Here's how the part is built. I have some questions about the finished solid (model axes, mm). A direction names the side the tool comes from. Round coordinates to 2 decimals unless told otherwise and drop trailing zeros. Order: outer loops, then holes, each group sorted by start corner. A loop starts at its lowest first (then second) coordinate and runs counter-clockwise, first axis right, second up. Notation, with made-up numbers: (29, 25) -> (68, 25) arc R34 cw to (68, 56) -> close; hole circle Ø4 at (-24, -37). An arc over 180 degrees is marked (long way). Use a Markdown table: item, result. Add a question column.
(1) I want a section at A-A, the plane y = 8.75. Please give me the cut outline in (x, z).
(2) Thinking about a two-plate mould opening in X: for faces 1 (the face through (-22, 6.65, 11)), 2 (the face through (13.14, 2.22, -10.1)), 3 (the face through (13.75, 9.69, 11.14)), which applies, pulls with the +X half, pulls with the -X half, needs draft (parallel to the pull), parting line crosses it, or undercut?
(3) I'm going to push flat-ended pins straight in: P1, Ø1.2, axis at y = 8.5, z = 4.5, coming from the +X side; P2, Ø1.8, axis at x = 10, z = 33, coming from the -Y side; P3, Ø2, axis at y = 10, z = 31.5, coming from the -X side. Where does each tip first touch, or does it pass through?
(4) I want a section at C-C, the plane x = -6. Please give me the cut outline in (y, z).
(5) On a 3-axis mill with a long thin cutter (end or side, diameter ignored), from which of +Z, -Z, +X, -X, +Y, -Y can I reach the whole of each face in a straight line? I mean faces 4 (the face through (11, 2, 35)), 5 (the face through (-18.75, 10, 4)), 6 (the face through (18.75, 10, 4)). Say none if no direction works.
(6) If I drill on probe 1 along X at (y, z) = (9.25, 32); probe 2 along X at (y, z) = (2, 11.25); probe 3 along Z at (x, y) = (-9.5, 2), over which ranges is the centre line in solid material (lowest first)?
(7) I want a section at B-B, the plane y = 1.25. Give the number of separate pieces and of enclosed holes in the cut face, then the cut area to 3 significant figures.
(8) I want a section at D-D, the plane x = 20. Please give me the cut outline in (y, z), then the cut area to 3 significant figures.
from build123d import *

# Parameters (mm, degrees)
SCHIZZO3_R                   = 2.25
ESTRUSIONE_ESTRUSIONE1_DEPTH = 12.65
SCHIZZO1_R                   = 3
TAGLIO_ESTRUSIONE1_DEPTH     = 4.5
SCHIZZO4_R                   = 10.75
SCHIZZO4_R_2                 = 1.45
TAGLIO_ESTRUSIONE2_DEPTH     = 48.529438246
SCHIZZO6_R                   = 5
TAGLIO_ESTRUSIONE3_DEPTH     = 6
SCHIZZO7_W                   = 16
SCHIZZO7_H                   = 77
TAGLIO_ESTRUSIONE4_DEPTH     = 6


with BuildPart() as part:
    # Schizzo3 → Estrusione-Estrusione1 (new body)
    with BuildSketch(Plane(origin=(0, 0, 0), x_dir=(1, 0, 0), z_dir=(0, 1, 0))):
        with BuildLine():
            Line((-24.75, 2.881082761), (-24.75, -25.381082761))
            ThreePointArc((-24.75, -25.381082761), (0, -39.75), (24.75, -25.381082761))
            Line((24.75, -25.381082761), (24.75, 2.881082761))
            ThreePointArc((24.75, 2.881082761), (0, 17.25), (-24.75, 2.881082761))
        make_face()
        with Locations(Location((-18.75, 2.75, 0), (0, 0, 270))):
            Circle(SCHIZZO3_R, mode=Mode.SUBTRACT)
        with Locations(Location((18.75, 2.75, 0), (0, 0, 90))):
            Circle(SCHIZZO3_R, mode=Mode.SUBTRACT)
        with Locations(Location((18.75, -25.25, 0), (0, 0, 270))):
            Circle(SCHIZZO3_R, mode=Mode.SUBTRACT)
        with Locations(Location((-18.75, -25.25, 0), (0, 0, 90))):
            Circle(SCHIZZO3_R, mode=Mode.SUBTRACT)
        with Locations(Location((-18.75, -11.25, 0), (0, 0, 270))):
            Circle(SCHIZZO3_R, mode=Mode.SUBTRACT)
        with Locations(Location((18.75, -11.25, 0), (0, 0, 90))):
            Circle(SCHIZZO3_R, mode=Mode.SUBTRACT)
    extrude(amount=ESTRUSIONE_ESTRUSIONE1_DEPTH)

    # Schizzo1 → Taglio-Estrusione1 (cut)
    with BuildSketch(Plane(origin=(0, 0, 0), x_dir=(1, 0, 0), z_dir=(0, 1, 0))):
        with Locations(Location((-11, -32, 0), (0, 0, 270))):
            Circle(SCHIZZO1_R)
        with Locations(Location((11, -32, 0), (0, 0, 90))):
            Circle(SCHIZZO1_R)
        with BuildLine():
            Line((-14, 8), (-14, -8))
            ThreePointArc((-14, -8), (-13.121320344, -10.121320344), (-11, -11))
            Line((-11, -11), (0, -11))
            Line((0, -11), (11, -11))
            ThreePointArc((11, -11), (13.121320344, -10.121320344), (14, -8))
            Line((14, -8), (14, 8))
            ThreePointArc((14, 8), (13.121320344, 10.121320344), (11, 11))
            Line((11, 11), (0, 11))
            Line((0, 11), (-11, 11))
            ThreePointArc((-11, 11), (-13.121320344, 10.121320344), (-14, 8))
        make_face()
    extrude(amount=TAGLIO_ESTRUSIONE1_DEPTH, mode=Mode.SUBTRACT)

    # Schizzo4 → Taglio-Estrusione2 (cut, through all)
    with BuildSketch(Plane.XZ.offset(-4.5)):
        with Locations(Location((0, 0, 0), (0, 0, 270))):
            Circle(SCHIZZO4_R)
        with Locations(Location((-11, 8, 0), (0, 0, 270))):
            Circle(SCHIZZO4_R_2)
        with Locations(Location((-11, -8, 0), (0, 0, 270))):
            Circle(SCHIZZO4_R_2)
        with Locations(Location((11, -8, 0), (0, 0, 270))):
            Circle(SCHIZZO4_R_2)
        with Locations(Location((11, 8, 0), (0, 0, 270))):
            Circle(SCHIZZO4_R_2)
        with Locations(Location((-11, 32, 0), (0, 0, 270))):
            Circle(SCHIZZO4_R_2)
        with Locations(Location((11, 32, 0), (0, 0, 270))):
            Circle(SCHIZZO4_R_2)
    extrude(amount=-TAGLIO_ESTRUSIONE2_DEPTH, mode=Mode.SUBTRACT)

    # Schizzo6 → Taglio-Estrusione3 (cut)
    with BuildSketch(Plane(origin=(0, 12.65, 0), x_dir=(1, 0, 0), z_dir=(0, 1, 0))):
        with Locations(Location((-18.75, 2.75, 0), (0, 0, 270))):
            Circle(SCHIZZO6_R)
        with Locations(Location((-18.75, -11.25, 0), (0, 0, 270))):
            Circle(SCHIZZO6_R)
        with Locations(Location((-18.75, -25.25, 0), (0, 0, 270))):
            Circle(SCHIZZO6_R)
        with Locations(Location((18.75, -25.25, 0), (0, 0, 270))):
            Circle(SCHIZZO6_R)
        with Locations(Location((18.75, -11.25, 0), (0, 0, 270))):
            Circle(SCHIZZO6_R)
        with Locations(Location((18.75, 2.75, 0), (0, 0, 270))):
            Circle(SCHIZZO6_R)
    extrude(amount=-TAGLIO_ESTRUSIONE3_DEPTH, mode=Mode.SUBTRACT)

    # Schizzo7 → Taglio-Estrusione4 (cut)
    with BuildSketch(Plane(origin=(0, 12.65, 0), x_dir=(1, 0, 0), z_dir=(0, 1, 0))):
        with Locations((-26.75, -11.25)):
            Rectangle(SCHIZZO7_W, SCHIZZO7_H)
        with Locations((26.75, -11.25)):
            Rectangle(SCHIZZO7_W, SCHIZZO7_H)
    extrude(amount=-TAGLIO_ESTRUSIONE4_DEPTH, mode=Mode.SUBTRACT)


solid = part.part
Taken from the geometry:
| question | item | result |
|---|---|---|
| 1 | outline | (-18.75, -10.21) arc R28.5 ccw to (18.75, -10.21) -> (18.75, -7.75) arc R5 cw to (18.75, 2.25) -> (18.75, 6.25) arc R5 cw to (18.75, 16.25) -> (18.75, 20.25) arc R5 cw to (18.75, 30.25) -> (18.75, 32.71) arc R28.5 ccw to (-18.75, 32.71) -> (-18.75, 30.25) arc R5 cw to (-18.75, 20.25) -> (-18.75, 16.25) arc R5 cw to (-18.75, 6.25) -> (-18.75, 2.25) arc R5 cw to (-18.75, -7.75) -> close; hole circle Ø2.9 at (-11, -8); hole circle Ø2.9 at (-11, 8); hole circle Ø2.9 at (-11, 32); hole circle Ø21.5 at (0, 0); hole circle Ø2.9 at (11, -8); hole circle Ø2.9 at (11, 8); hole circle Ø2.9 at (11, 32) |
| 2 | face 1 | needs draft |
| 2 | face 2 | undercut |
| 2 | face 3 | pulls with the +X half |
| 3 | P1 | stops at x = 18.75 |
| 3 | P2 | stops at y = 4.5 |
| 3 | P3 | stops at x = -18.75 |
| 4 | outline | (0, -16.61) -> (12.65, -16.61) -> (12.65, -8.92) -> (4.5, -8.92) -> (4.5, -11) -> (0, -11) -> close; (0, 11) -> (4.5, 11) -> (4.5, 8.92) -> (12.65, 8.92) -> (12.65, 39.11) -> (0, 39.11) -> close |
| 5 | face 4 | -Y |
| 5 | face 5 | +Z, -Z, -X, +Y |
| 5 | face 6 | +Z, -Z, +X, +Y |
| 6 | probe 1 | x = -18.75 to -12.45, -9.55 to 9.55, 12.45 to 18.75 |
| 6 | probe 2 | x = -24.75 to -21, -16.5 to 16.5, 21 to 24.75 |
| 6 | probe 3 | z = -15.62 to -11, 11 to 29.4, 34.6 to 38.12 |
| 7 | separate pieces | 1 |
| 7 | enclosed holes | 9 |
| 7 | area | 1,650 mm2 |
| 8 | outline | (0, -9.05) -> (6.65, -9.05) -> (6.65, -4.62) -> (0, -4.62) -> close; (0, -0.88) -> (6.65, -0.88) -> (6.65, 9.38) -> (0, 9.38) -> close; (0, 13.12) -> (6.65, 13.12) -> (6.65, 23.38) -> (0, 23.38) -> close; (0, 27.12) -> (6.65, 27.12) -> (6.65, 31.55) -> (0, 31.55) -> close |
| 8 | area | 195 mm2 |
